CAD build for the part. Positions are in the model's coordinates, mm. A direction names the side the tool comes from. Coordinates: 2 decimals unless noted, no trailing zeros. Order: outer loops, then holes, each group sorted by start corner. A loop starts at its lowest first (then second) coordinate and runs counter-clockwise, first axis right, second up.
from build123d import *

# Parameters (mm, degrees)
BOSS_EXTRUDE1_DEPTH = 6.604
FILLET1_R           = 12.7
CUT_EXTRUDE1_REACH  = 8.604
CUT_EXTRUDE2_DEPTH  = 7.604
SKETCH5_W           = 6.35
SKETCH5_H           = 6.35
BOSS_EXTRUDE2_DEPTH = 6.604


with BuildPart() as part:
    # Sketch1 → Boss-Extrude1 (new body)
    with BuildSketch(Plane(origin=(0, 0, 0), x_dir=(1, 0, 0), z_dir=(0, 1, 0))):
        Polygon((-152.4, -38.1), (-152.4, -69.85), (0, -69.85), (0, 0), (-31.75, 0), (-31.75, -38.1), align=None)
    extrude(amount=BOSS_EXTRUDE1_DEPTH)

    # Fillet1
    fillet1_edges = [part.edges().sort_by_distance(p)[0] for p in [
        (-152.4, 3.302, 69.85),
        (-152.4, 3.302, 38.1),
        (-31.75, 3.302, 38.1),
        (-31.75, 3.302, 0),
    ]]
    fillet(fillet1_edges, radius=FILLET1_R)

    # Sketch2 → Cut-Extrude1 (cut, up to next)
    with BuildSketch(Plane(origin=(0, 6.604, 0), x_dir=(1, 0, 0), z_dir=(0, 1, 0)), mode=Mode.PRIVATE) as cut_extrude1_sk1:
        with BuildLine():
            Line((-127, -57.4675), (-25.4, -57.4675))
            ThreePointArc((-25.4, -57.4675), (-21.9075, -53.975), (-25.4, -50.4825))
            Line((-25.4, -50.4825), (-127, -50.4825))
            ThreePointArc((-127, -50.4825), (-130.4925, -53.975), (-127, -57.4675))
        make_face()
    cut_extrude1_tool1 = extrude(cut_extrude1_sk1.sketch, amount=-CUT_EXTRUDE1_REACH, mode=Mode.PRIVATE) & part.part
    add(cut_extrude1_tool1.solids().sort_by_distance((-76.2, 6.604, 53.975))[0], mode=Mode.SUBTRACT)

    # Sketch4 → Cut-Extrude2 (cut, through all)
    with BuildSketch(Plane(origin=(0, 6.604, 0), x_dir=(1, 0, 0), z_dir=(0, 1, 0))):
        Polygon((0, -16.9672), (-6.35, -16.9672), (-6.35, -14.6812), (-12.2936, -14.6812), (-12.2936, -16.9672), (-13.97, -16.9672), (-13.97, -21.1328), (-12.2936, -21.1328), (-12.2936, -23.4188), (-6.35, -23.4188), (-6.35, -21.1328), (0, -21.1328), align=None)
        Polygon((0, -36.0172), (-6.35, -36.0172), (-6.35, -33.7312), (-12.2936, -33.7312), (-12.2936, -36.0172), (-13.97, -36.0172), (-13.97, -40.1828), (-12.2936, -40.1828), (-12.2936, -42.4688), (-6.35, -42.4688), (-6.35, -40.1828), (0, -40.1828), align=None)
    extrude(amount=-CUT_EXTRUDE2_DEPTH, mode=Mode.SUBTRACT)

    # Sketch5 → Boss-Extrude2 (add)
    with BuildSketch(Plane(origin=(0, 6.604, 0), x_dir=(1, 0, 0), z_dir=(0, 1, 0))):
        with Locations((3.175, -9.525)):
            Rectangle(SKETCH5_W, SKETCH5_H)
        with Locations((3.175, -28.575)):
            Rectangle(SKETCH5_W, SKETCH5_H)
        with Locations((3.175, -47.625)):
            Rectangle(SKETCH5_W, SKETCH5_H)
    extrude(amount=-BOSS_EXTRUDE2_DEPTH)


solid = part.part
1) Which spindle directions (+Z, -Z, +X, -X, +Y, -Y) get a long thin tool onto all of the face, cutting with end or side? Do faces 5 (the flat face through (0, 3, 23)), 6 (the flat face through (-31.75, 3, 19)), 7 (the cylindrical face through (-21.91, 3.35, 54.05)). Say none if no direction does.
2) Slice it at A-A (x = -47). List the corners of the cut face in (y, z).
3) Two-plate mould, pull along Z, no slides. Class faces 1 (the cylindrical face through (-148.78, 3.35, 66.03)), 2 (the flat face through (3, 3, 6.35)), 3 (the flat face through (6.35, 3, 48)), 4 (the flat face through (-13.97, 3, 38)): released by +Z, released by -Z, zero draft, split by the parting line, or undercut.
4) Slice it at B-B (z = 54.5). List the corners of the cut face in (x, y), plus the area to 3 significant figures.
5) Pin check, flat tips, straight feed: P1, Ø1, axis at y = 6, z = 13.5, coming from the -X side; P2, Ø1.2, axis at y = 3, z = 19, coming from the +X side; P3, Ø3, axis at x = -49.5, y = 1, coming from the -Z side. Stop position of each tip, or through.
6) Drill centre lines: probe 1 along Z at (x, y) = (-4.5, 2); probe 2 along Z at (x, y) = (-6.5, 0.75); probe 3 along Z at (x, y) = (-111, 0.5). Where is each one in solid material? Low to high.
7) Slice it at C-C (z = 19). List the corners of the cut face in (x, y), plus the area to 3 significant figures.
Worked out:
1. face 5: +X, +Y, -Y
1. face 6: -Z, -X, +Y, -Y
1. face 7: +Y, -Y
2. outline: (0, 38.1) - (6.6, 38.1) - (6.6, 50.48) - (0, 50.48) - close; (0, 57.47) - (6.6, 57.47) - (6.6, 69.85) - (0, 69.85) - close
3. face 1: released by +Z
3. face 2: released by -Z
3. face 3: zero draft
3. face 4: undercut
4. outline: (-152.4, 0) - (-130.45, 0) - (-130.45, 6.6) - (-152.4, 6.6) - close; (-21.95, 0) - (0, 0) - (0, 6.6) - (-21.95, 6.6) - close
4. area: 290 mm2
5. P1: stops at x = -31.75
5. P2: stops at x = -13.97
5. P3: stops at z = 38.1
6. probe 1: z = 0 to 16.97, 21.13 to 36.02, 40.18 to 69.85
6. probe 2: z = 0 to 14.68, 23.42 to 33.73, 42.47 to 69.85
6. probe 3: z = 38.1 to 50.48, 57.47 to 69.85
7. outline: (-31.75, 0) - (-13.97, 0) - (-13.97, 6.6) - (-31.75, 6.6) - close
7. area: 117 mm2
